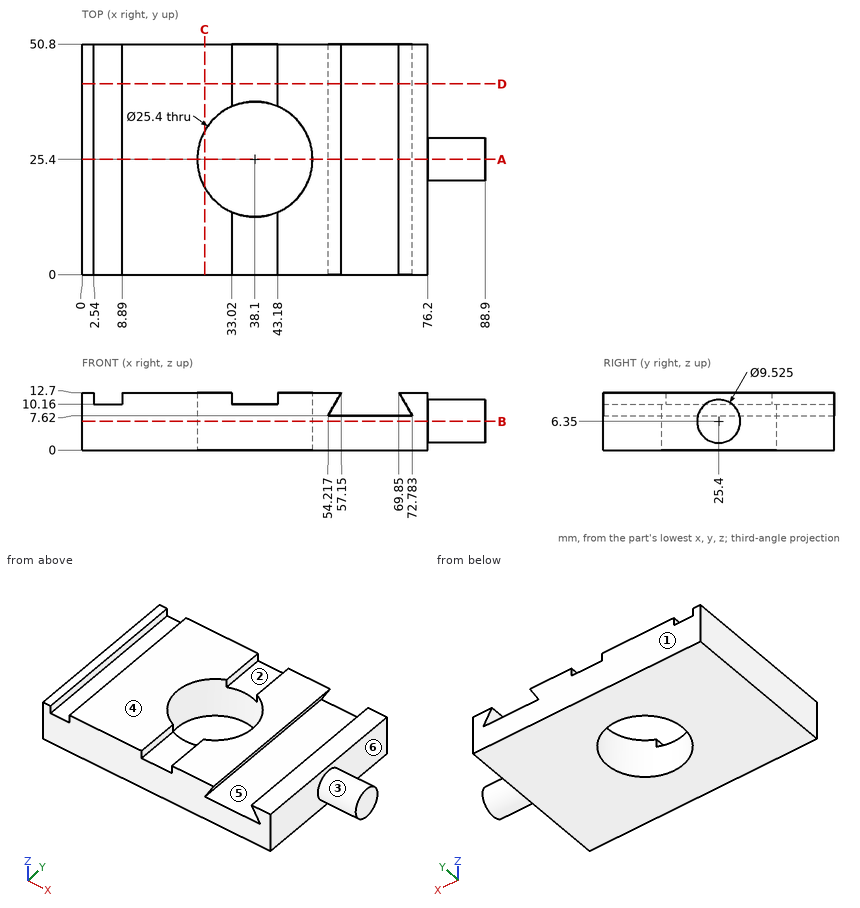
Print and shaded views of the part. All mm, measured from the part's lowest x, y and z. A direction names the side the tool comes from. Give positions to 0.01 mm unless a question says otherwise; leave off trailing zeros. Loops run counter-clockwise (first coordinate to the right, second up) from the corner with the lowest first, then second, coordinate; pieces in that order, holes last. Notation, with made-up numbers: (-25, 40) - (34, 40) arc R20 ccw to (34, 48) - close; hole circle Ø8 at (20.5, 74). An arc over 180 degrees is marked (long way). One line per item, written item: value. Start each with the question number.
1. Slice it at D-D (y = 42). List the corners of the cut face in (x, z), plus the area to 3 significant figures.
2. Pin check, flat tips, straight feed: pin 1 (8 mm diameter, centred on x = 36, y = 6, fed in from +Z); pin 2 (1.3 mm diameter, centred on y = 44.5, z = 11, fed in from +X); pin 3 (5.5 mm diameter, centred on x = 67, y = 25.5, fed in from +Z); pin 4 (8 mm diameter, centred on x = 38.5, y = 47, fed in from +Z). Stop position of each tip, or through.
3. Probe L1, parallel to Y at x = 38.1, z = 8; L2, parallel to X at y = 25.4, z = 9.5; L3, parallel to X at y = 25.4, z = 9.75. List the from-to ranges inside material, lowest first. Write a range as from..to.
4. Which spindle directions (+Z, -Z, +X, -X, +Y, -Y) get a long thin tool onto all of the face, cutting with end or side? Do the marked faces 1, 2 and 3. Say none if no direction does.
5. Slice it at A-A (y = 25.4). List the corners of the cut face in (x, z), plus the area to 3 significant figures.
6. Slice it at C-C (x = 27). List the corners of the cut face in (y, z).
7. Slice it at B-B (z = 6.35). List the corners of the cut face in (x, y), plus the area to 3 significant figures.
8. Pull direction X, two halves, no side cores. Call the marked faces 4, 5 and 6: pulls with the +X half, pulls with the -X half, needs draft (parallel to the pull), parting line crosses it, or undercut.
Solution:
1. outline: (0, 0) - (76.2, 0) - (76.2, 12.7) - (69.85, 12.7) - (72.78, 7.62) - (54.22, 7.62) - (57.15, 12.7) - (43.18, 12.7) - (43.18, 10.16) - (33.02, 10.16) - (33.02, 12.7) - (8.89, 12.7) - (8.89, 10.16) - (2.54, 10.16) - (2.54, 12.7) - (0, 12.7) - close
1. area: 846 mm^2
2. pin 1: stops at z = 12.7
2. pin 2: stops at x = 76.2
2. pin 3: stops at z = 7.62
2. pin 4: stops at z = 10.16
3. L1: y = 0..12.7, 38.1..50.8
3. L2: x = 0..25.4, 50.8..55.3, 71.7..88.9
3. L3: x = 0..25.4, 50.8..55.45, 71.55..88.9
4. face 1: +Z, -Z, +X, -X, +Y
4. face 2: +Z, +Y, -Y
4. face 3: +X
5. outline: (0, 0) - (25.4, 0) - (25.4, 12.7) - (8.89, 12.7) - (8.89, 10.16) - (2.54, 10.16) - (2.54, 12.7) - (0, 12.7) - close; (50.8, 0) - (76.2, 0) - (76.2, 1.59) - (88.9, 1.59) - (88.9, 11.11) - (76.2, 11.11) - (76.2, 12.7) - (69.85, 12.7) - (72.78, 7.62) - (54.22, 7.62) - (57.15, 12.7) - (50.8, 12.7) - close
5. area: 671 mm^2
6. outline: (0, 0) - (19.23, 0) - (19.23, 12.7) - (0, 12.7) - close; (31.57, 0) - (50.8, 0) - (50.8, 12.7) - (31.57, 12.7) - close
7. outline: (0, 0) - (76.2, 0) - (76.2, 20.64) - (88.9, 20.64) - (88.9, 30.16) - (76.2, 30.16) - (76.2, 50.8) - (0, 50.8) - close; hole circle Ø25.4 at (38.1, 25.4)
7. area: 3,490 mm^2
8. face 4: needs draft
8. face 5: undercut
8. face 6: pulls with the +X half
